Read the model definition and answer for the solid it produces. Units are mm, in the model's axes. A direction names the side the tool comes from. Coordinates: 2 decimals unless noted, no trailing zeros. Write each loop counter-clockwise with the first axis right and the second up, starting at its lowest first coordinate (ties: lowest second). Pieces come first, ordered by that corner, then holes. Notation, with made-up numbers: (5, 19) -> (10, 19) arc R18 ccw to (10, 51) -> close; hole circle Ø11 at (88.25, 45). An arc over 180 degrees is marked (long way). Answer in a Markdown table with one row per item. Add a question column.
Item 1: Given pin 1 Ø5 at (x, y) = (-3.5, 2) entering from +Z; pin 2 Ø0.5 at (x, z) = (12.5, 0.5) entering from +Y; pin 3 Ø2 at (x, y) = (-2.5, 27) entering from +Z, each flat-ended and moving along its own axis, determine where each tip first touches the part or whether it passes through.
Item 2: For a pull along X with two mould halves and no side action, classify faces 3 (the face through (33.65, 33.42, 0.49)), 4 (the face through (-13.948, 14.656, 0.493)), 5 (the face through (5, 5, 0)) as +X half, -X half, draft (parallel to the pull), parting line (faces both ways), or undercut.
Item 3: Straight lines are drawn through the part: line 1 (X direction, y = -13, z = 0.3); line 2 (Y direction, x = -23.5, z = 0.6); line 3 (Y direction, x = -1.5, z = 0.5). For each, find the intervals that lie inside material, in ascending order. Write a range as from..to.
Item 4: Section B-B on y = 13.5 is taken. Write down the section's boundary in (x, z).
Item 5: Which of the six approach directions +Z, -Z, +X, -X, +Y, -Y give full straight-line access (tool end or side, diameter ignored) to faces 1 (the face through (5, 5, 1)), 2 (the face through (13.589, 12.881, 0.493))?
Item 6: Section C-C on x = -20.5 is taken. Write down the section's boundary in (y, z).
Item 7: Section A-A on z = 0.6 is taken. Write down the section's boundary in (x, y), then the cut area to 3 significant figures.
```python
from build123d import *

# Parameters (mm, degrees)
F0_R     = 3.999999
F1_DEPTH = 1


with BuildPart() as f1:
    # F0 (on Top) → F1 (new body)
    with BuildSketch(Plane.XY):
        with BuildLine():
            Line((25, 30), (-30, 30))
            Line((-30, 30), (-30, -30))
            Line((-30, -30), (30, -30))
            Line((30, -30), (30, 25))
            ThreePointArc((30, 25), (33.535534, 33.535534), (25, 30))
        make_face()
        Polygon((28.292893, -29), (-28.292893, -29), (0, -0.707107), align=None, mode=Mode.SUBTRACT)
        Polygon((-29, -28.292893), (-29, 28.292893), (-0.707107, 0), align=None, mode=Mode.SUBTRACT)
        with BuildLine():
            Line((0.707107, 0), (26.835742, 26.128635))
            ThreePointArc((26.835742, 26.128635), (27.855411, 25.483282), (29, 25.101021))
            Line((29, 25.101021), (29, -28.292893))
            Line((29, -28.292893), (0.707107, 0))
        make_face(mode=Mode.SUBTRACT)
        with BuildLine():
            Line((0, 0.707107), (-28.292893, 29))
            Line((-28.292893, 29), (25.101021, 29))
            ThreePointArc((25.101021, 29), (25.483282, 27.855411), (26.128635, 26.835742))
            Line((26.128635, 26.835742), (0, 0.707107))
        make_face(mode=Mode.SUBTRACT)
        with Locations((30, 30)):
            Circle(F0_R, mode=Mode.SUBTRACT)
    extrude(amount=F1_DEPTH)


solid = f1.part
```
Results below:
| question | item | result |
|---|---|---|
| 1 | pin 1 | stops at z = 1 |
| 1 | pin 2 | stops at y = 30 |
| 1 | pin 3 | passes through |
| 2 | face 3 | parting line |
| 2 | face 4 | undercut |
| 2 | face 5 | draft |
| 3 | line 1 | x = -30..-29, -13.71..-12.29, 12.29..13.71, 29..30 |
| 3 | line 2 | y = -30..-29, -24.21..-22.79, 22.79..24.21, 29..30 |
| 3 | line 3 | y = -30..-29, -2.21..-0.79, 0.79..2.21, 29..30 |
| 4 | outline | (-30, 0) -> (-29, 0) -> (-29, 1) -> (-30, 1) -> close; (-14.21, 0) -> (-12.79, 0) -> (-12.79, 1) -> (-14.21, 1) -> close; (12.79, 0) -> (14.21, 0) -> (14.21, 1) -> (12.79, 1) -> close; (29, 0) -> (30, 0) -> (30, 1) -> (29, 1) -> close |
| 5 | face 1 | +Z, +X, -X, +Y, -Y |
| 5 | face 2 | +Z, -Z |
| 6 | outline | (-30, 0) -> (-29, 0) -> (-29, 1) -> (-30, 1) -> close; (-21.21, 0) -> (-19.79, 0) -> (-19.79, 1) -> (-21.21, 1) -> close; (19.79, 0) -> (21.21, 0) -> (21.21, 1) -> (19.79, 1) -> close; (29, 0) -> (30, 0) -> (30, 1) -> (29, 1) -> close |
| 7 | outline | (-30, -30) -> (30, -30) -> (30, 25) arc R5 ccw (long way) to (25, 30) -> (-30, 30) -> close; hole (-29, -28.29) -> (-0.71, 0) -> (-29, 28.29) -> close; hole (-28.29, -29) -> (28.29, -29) -> (0, -0.71) -> close; hole (-28.29, 29) -> (0, 0.71) -> (26.13, 26.84) arc R5 cw to (25.1, 29) -> close; hole (0.71, 0) -> (29, -28.29) -> (29, 25.1) arc R5 cw to (26.84, 26.13) -> close; hole circle Ø8 at (30, 30) |
| 7 | area | 414 mm2 |
